Input: dimensioned drawing with shaded views. Units: mm. Origin: part minimum x, y, z. A direction names the side the tool comes from. Give positions to 0.01 mm unless a question says otherwise; leave off trailing zeros. Loops run counter-clockwise (first coordinate to the right, second up) from the corner with the lowest first, then second, coordinate; pieces in that order, holes last. Notation, with made-up numbers: M 40,57 L 56,57 A29 cw 56,81 Z; hole C 89,61.25 d8. An arc over 180 degrees is marked long. Answer in a Markdown table with one row per item.
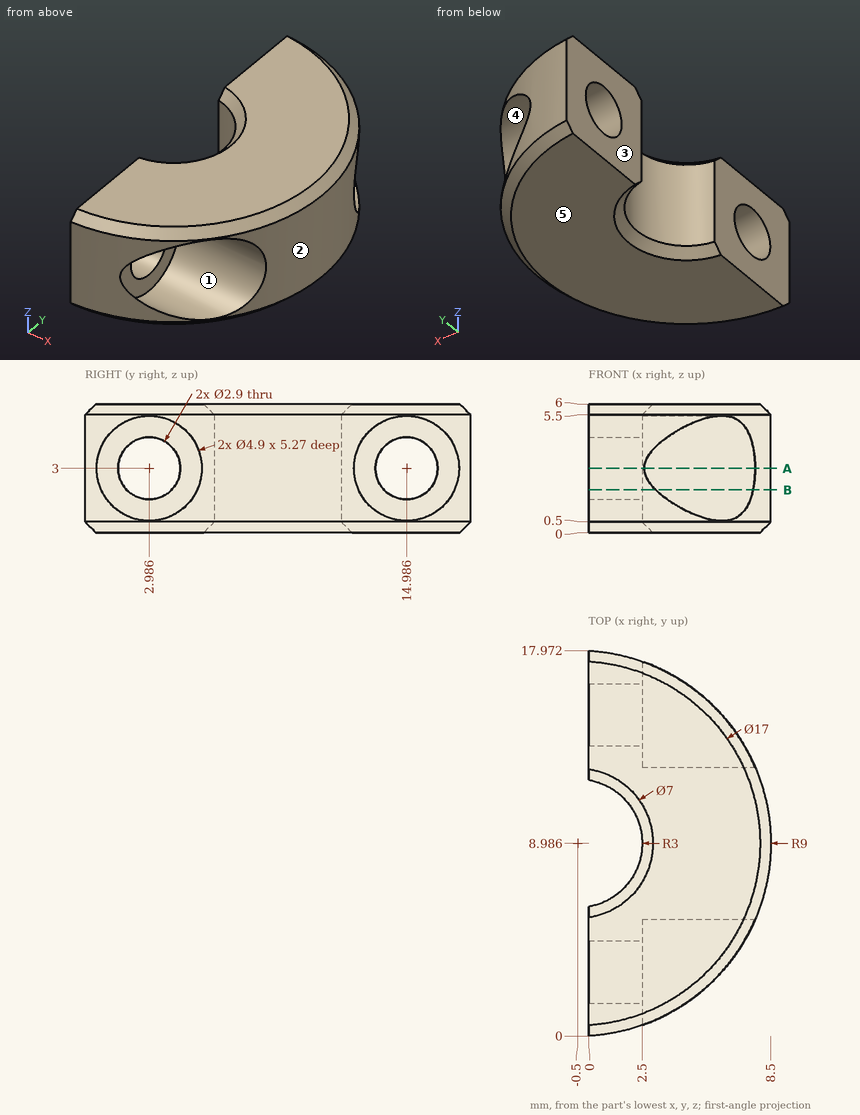
Q1. Ray query, probe 1 along X at (y, z) = (15, 5); probe 2 along Z at (x, y) = (5.75, 13.75) (1 decimal); probe 3 along Z at (x, y) = (1.75, 14.5). Return the intervals inside material, ascending. Write a range as from..to.
Values follow:
| item | result |
|---|---|
| probe 1 | 0..2.5 |
| probe 2 | 0..0.9, 5.1..6 |
| probe 3 | 0..1.63, 4.37..6 |
Q2. Reachability of the marked faces 1 and 2 from +Z, -Z, +X, -X, +Y, -Y: full face, straight path, thin tool, end or side. Return the list, or none.
Values follow:
| item | result |
|---|---|
| face 1 | +X |
| face 2 | +Z, -Z, +X |
Q3. Section query B-B (z = 2). Give the number of separate pieces and of enclosed holes in the cut face.
Values follow:
| item | result |
|---|---|
| separate pieces | 3 |
| enclosed holes | 0 |
Q4. Mould query, pull axis Z, two halves, no side actions, for the marked faces 3, 4 and 5. Classes: +Z half, -Z half, draft (parallel to the pull), parting line (faces both ways), or undercut.
Values follow:
| item | result |
|---|---|
| face 3 | draft |
| face 4 | undercut |
| face 5 | -Z half |
Q5. Section query A-A (z = 3). Output: boundary loops of the cut face in (x, y).
Values follow:
| item | result |
|---|---|
| outline | M 0,0 A9 ccw 2.6,0.54 L 2.5,0.54 L 2.5,1.54 L 0,1.54 Z; M 0,4.44 L 2.5,4.44 L 2.5,5.44 L 7.77,5.44 A9 ccw 7.77,12.54 L 2.5,12.54 L 2.5,13.54 L 0,13.54 L 0,11.94 A3 cw 0,6.03 Z; M 0,16.44 L 2.5,16.44 L 2.5,17.44 L 2.6,17.44 A9 ccw 0,17.97 Z |
Q6. Contact query for flat-ended pins moving along their axis: pin 1 Ø1.5 at (x, z) = (3, 2) entering from -Y; pin 2 Ø1.5 at (x, z) = (4, 2.5) entering from +Y; pin 3 Ø1.5 at (y, z) = (7.5, 2.5) entering from -X. Output: stop coordinate, or through.
Values follow:
| item | result |
|---|---|
| pin 1 | y = 0.42 |
| pin 2 | y = 12.88 |
| pin 3 | x = 1.5 |
